from build123d import *

# Parameters (mm, degrees)
BASE_DEPTH      = 2743.2
SKETCH2_W       = 304.8
SKETCH2_H       = 76.2
LEFT_SLOT_DEPTH = 2752.653640995
LEFT_CUT_DEPTH  = 152.4


with BuildPart() as part:
    # Sketch1 → Base (new body)
    with BuildSketch(Plane(origin=(0, 0, 0), x_dir=(0, 0, -1), z_dir=(1, 0, 0))):
        with BuildLine():
            Line((152.4, 0), (-152.4, 0))
            ThreePointArc((-152.4, 0), (0, -152.4), (152.4, 0))
        make_face()
    extrude(amount=BASE_DEPTH)

    # Sketch2 → Left Slot (cut, symmetric)
    with BuildSketch(Plane.XY):
        with Locations((457.2, -114.3)):
            Rectangle(SKETCH2_W, SKETCH2_H)
    left_slot = extrude(amount=LEFT_SLOT_DEPTH, both=True, mode=Mode.SUBTRACT)

    # Right Slot: Left Slot across plane
    add(left_slot.mirror(Plane(origin=(1371.6, 0, 0), x_dir=(0, 0, 1), z_dir=(1, 0, 0))), mode=Mode.SUBTRACT)

    # Sketch3 → Left Cut (cut)
    with BuildSketch(Plane.ZY):
        with BuildLine():
            Line((152.4, 0), (-152.4, 0))
            ThreePointArc((-152.4, 0), (0, -152.4), (152.4, 0))
        make_face()
    left_cut = extrude(amount=-LEFT_CUT_DEPTH, mode=Mode.SUBTRACT)

    # Right Cut: Left Cut across plane
    add(left_cut.mirror(Plane(origin=(1371.6, 0, 0), x_dir=(0, 0, 1), z_dir=(1, 0, 0))), mode=Mode.SUBTRACT)


solid = part.part
Build history of the part. All positions in model axes, mm. A direction names the side the tool comes from. Coordinates: 2 decimals unless noted, no trailing zeros. Write each loop counter-clockwise with the first axis right and the second up, starting at its lowest first coordinate (ties: lowest second). Pieces come first, ordered by that corner, then holes.
(1) Cut at B-B on y = -120.5. List the corners of the cut face in (x, z), and give its area (3 significant figures).
(2) Mould opens along X. For faces 1 (the flat face through (2590.8, -58, -2)), 2 (the flat face through (152.4, -58, -2)), 3 (the flat face through (304.8, -106, 2)), 4 (the flat face through (1355, 0, -2)) say: pulls with the +X half, pulls with the -X half, needs draft (parallel to the pull), parting line crosses it, or undercut.
(3) Pin check, flat tips, straight feed: pin 1 Ø1 at (x, z) = (1183, -59.5) entering from -Y; pin 2 Ø3 at (x, y) = (595, -64.5) entering from -Z; pin 3 Ø1 at (x, y) = (755.5, -103.5) entering from +Z. Stop position of each tip, or through.
(4) 3-axis set-ups, long thin cutter, end or side, ignore diameter. For faces 5 (the flat face through (2288, -76.2, 2)), 6 (the cylindrical face through (1354.531, -152.363, 3.351)): which of +Z, -Z, +X, -X, +Y, -Y reach the whole face in a straight line?
(5) Cut at A-A on z = 0. List the corners of the cut face in (x, y).
(6) Drill centre lines: line 1 (X direction, y = -118.5, z = 90); line 2 (Y direction, x = 2232.5, z = 40); line 3 (Y direction, x = 1533, z = 43.5). Where is each one in solid material? Low to high.
(7) Cut at C-C on x = 761.5. List the corners of the cut face in (y, z), and give its area (3 significant figures).
Working result:
1. outline: (152.4, -93.3) - (304.8, -93.3) - (304.8, 93.3) - (152.4, 93.3) - close; (609.6, -93.3) - (2133.6, -93.3) - (2133.6, 93.3) - (609.6, 93.3) - close; (2438.4, -93.3) - (2590.8, -93.3) - (2590.8, 93.3) - (2438.4, 93.3) - close
1. area: 341,000 mm2
2. face 1: pulls with the +X half
2. face 2: pulls with the -X half
2. face 3: undercut
2. face 4: needs draft
3. pin 1: stops at y = -140.52
3. pin 2: stops at z = -138.77
3. pin 3: stops at z = 112.32
4. face 5: +Z, -Z, -Y
4. face 6: +X, -X, -Y
5. outline: (152.4, -152.4) - (304.8, -152.4) - (304.8, -76.2) - (609.6, -76.2) - (609.6, -152.4) - (2133.6, -152.4) - (2133.6, -76.2) - (2438.4, -76.2) - (2438.4, -152.4) - (2590.8, -152.4) - (2590.8, 0) - (152.4, 0) - close
6. line 1: x = 152.4 to 304.8, 609.6 to 2133.6, 2438.4 to 2590.8
6. line 2: y = -76.2 to 0
6. line 3: y = -146.06 to 0
7. outline: (0, -152.4) - (0, 152.4) arc R152.4 ccw to start
7. area: 36,500 mm2
